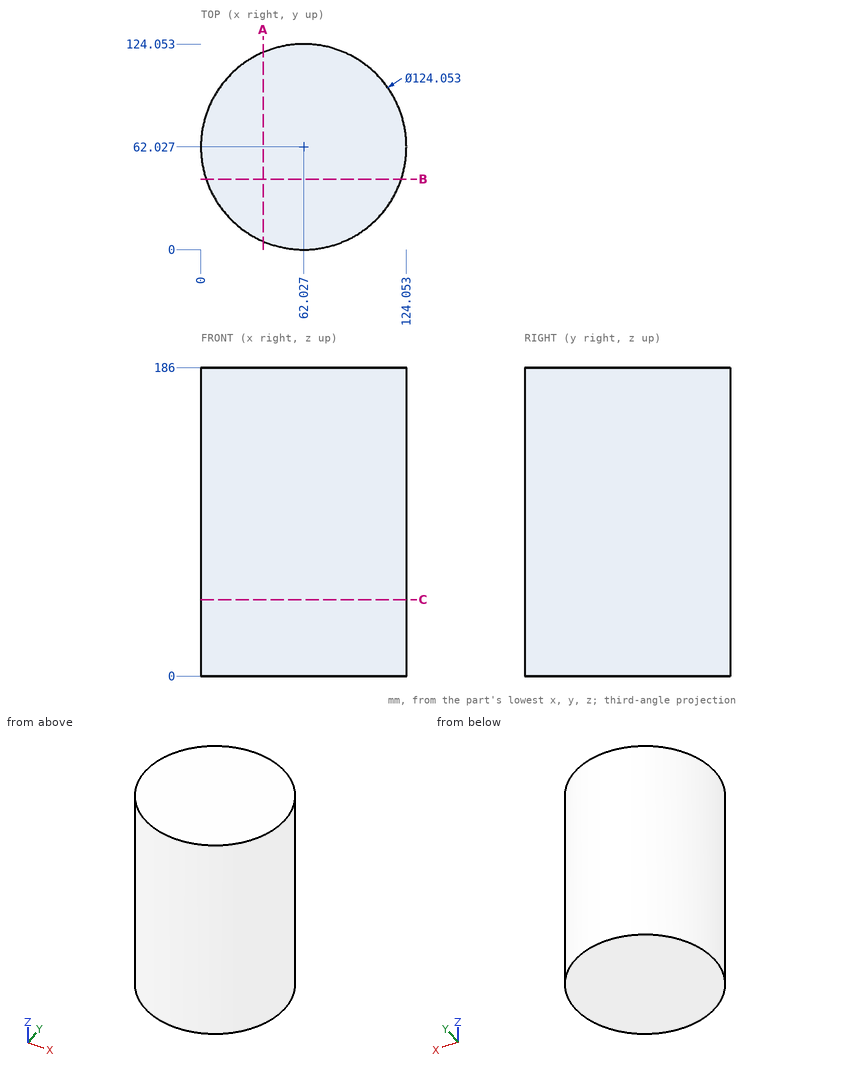
For this review, use the dimensioned drawing (mm, ordinates from the lowest corner) and the shaded views. Give positions to 0.01 mm unless a question says otherwise; leave off trailing zeros. Order: outer loops, then holes, each group sorted by start corner. A loop starts at its lowest first (then second) coordinate and runs counter-clockwise, first axis right, second up. Notation, with made-up numbers: M 7,-10.75 L 11,-10.75 A15 ccw 11,2.25 Z; hole C -31,14.25 d4. An arc over 180 degrees is marked long. One line per question, with ' | ' between items. Start each with the question number.
1) Wall thickness on L1, parallel to Y at x = 60, z = 136; L2, parallel to X at y = 61.5, z = 135.5; L3, parallel to X at y = 81.5, z = 74: over which ranges is each line inside the solid? List them lowest first. Write a range as from..to.
2) Consider section A-A, the plane x = 37.5. Give the boundary of the cut face in (y, z) (1 decimal), then the cut area to 3 significant figures.
3) Consider section C-C, the plane z = 46. Give the boundary of the cut face in (x, y).
4) Clearance check with flat-ended pins moving along their axes: P1, Ø10, axis at x = 36, z = 117.5, coming from the +Y side; P2, Ø8, axis at y = 47, z = 129.5, coming from the +X side (1 decimal); P3, Ø1.5, axis at y = 71, z = 150.5, coming from the -X side. State where each tip first meets the part, or that it passes through.
5) Consider section B-B, the plane y = 42.5. Give the boundary of the cut face in (x, z).
Found:
1) L1: y = 0.03..124.02 | L2: x = 0..124.05 | L3: x = 3.14..120.92
2) outline: M 5.1,0 L 119,0 L 119,186 L 5.1,186 Z | area: 21,200 mm²
3) outline: C 62.03,62.03 d124.05
4) P1: stops at y = 120.38 | P2: stops at x = 123.1 | P3: stops at x = 0.55
5) outline: M 3.15,0 L 120.9,0 L 120.9,186 L 3.15,186 Z
